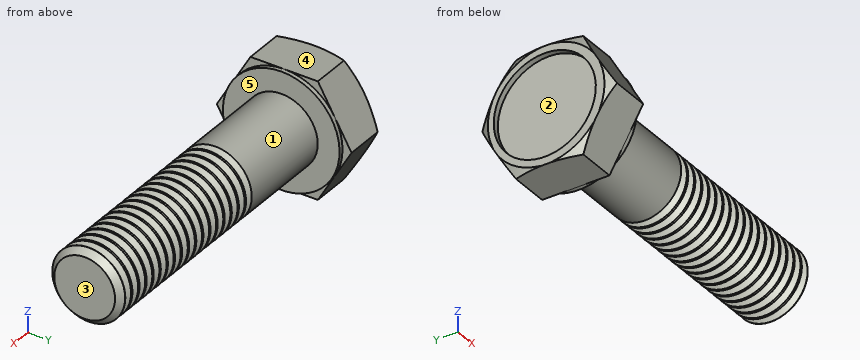
```python
from build123d import *

# Parameters (mm, degrees)
BASEHEAD_DEPTH     = 6.63
INDENT_START       = -0.82875
INDENT_2_OUTLINE_R = 7
INDENT_2_DEPTH     = 0.82875
SKETCH4_W          = 0.6
SKETCH4_H          = 11.237604307
THDSCHPAT_COUNT    = 18
THDSCHPAT_PITCH    = 1.444444444


# Read off the part's stored shape, not the designer's step: Indent
with BuildPart() as part:
    # Sketch1 → BaseHead (new body)
    with BuildSketch(Plane(origin=(0, 0, 0), x_dir=(0, 0, -1), z_dir=(1, 0, 0))):
        Polygon((8, 4.618802154), (8, -4.618802154), (0, -9.237604307), (-8, -4.618802154), (-8, 4.618802154), (0, 9.237604307), align=None)
    extrude(amount=BASEHEAD_DEPTH)

    # Indent outline → Indent (revolve)
    with BuildSketch(Plane.YX):
        Polygon((5, 6.63), (5, 45.802), (4.172, 46.63), (0, 46.63), (0, 6.63), align=None)
    revolve(axis=Axis((0, 0, 0), (1, 0, 0)))

    # Indent 2 outline → Indent 2 (cut)
    with BuildSketch(Plane.ZY.offset(INDENT_START)):
        with Locations((0.033212245, 0.192376607)):
            Circle(INDENT_2_OUTLINE_R)
    extrude(amount=INDENT_2_DEPTH, mode=Mode.SUBTRACT)

    # Sketch3 → HeadChamfer (revolve, cut)
    with BuildSketch(Plane.XY, mode=Mode.PRIVATE) as headchamfer_sk:
        Polygon((0, 8), (3.601282526, 14.237604307), (3.601282526, 19.237604307), (-10, 19.237604307), (-10, 8), align=None)
    revolve(headchamfer_sk.sketch.rotate(Axis((0, 0, 0), (1, 0, 0)), 90), axis=Axis((0, 0, 0), (1, 0, 0)), mode=Mode.SUBTRACT)

    # Sketch4 → BearingFace (revolve, cut)
    with BuildSketch(Plane.XY, mode=Mode.PRIVATE) as bearingface_sk:
        with Locations((6.33, 13.618802154)):
            Rectangle(SKETCH4_W, SKETCH4_H)
    revolve(bearingface_sk.sketch.rotate(Axis((0, 0, 0), (1, 0, 0)), 90), axis=Axis((0, 0, 0), (1, 0, 0)), mode=Mode.SUBTRACT)

    # ThdSchSke → ThreadSchematic (revolve, cut)
    with BuildSketch(Plane.XY):
        Polygon((20.63, -4.172), (20.050228158, -5), (20.050228158, -6.25), (21.209771842, -6.25), (21.209771842, -5), align=None)
    threadschematic = revolve(axis=Axis((-3.175, 0, 0), (1, 0, 0)), mode=Mode.SUBTRACT)

    # ThdSchPat: ThreadSchematic ×18
    with Locations(*[(i * THDSCHPAT_PITCH, 0, 0) for i in range(1, THDSCHPAT_COUNT)]):
        add(threadschematic, mode=Mode.SUBTRACT)


solid = part.part
```
Build history of the part. All positions in model axes, mm. Face numbers are marked on the shaded views. A direction names the side the tool comes from. Coordinates: 2 decimals unless noted, no trailing zeros. Order: outer loops, then holes, each group sorted by start corner. A loop starts at its lowest first (then second) coordinate and runs counter-clockwise, first axis right, second up. Notation, with made-up numbers: M 51.25,81 L 109.25,81 A18 ccw 109.25,90 Z; hole C 30,24 d6. An arc over 180 degrees is marked long. One line per question, with ' | ' between items. Start each with the question number.
1. Cut at A-A (x = 13.5). Write the cut outline in (y, z).
2. Tool access for the marked faces 4 and 5: list every direction of +Z, -Z, +X, -X, +Y, -Y with a clear straight run to the whole face (end or side of a thin tool).
3. Wall check: line 1 along X through (y, z) = (-6, -0.5); line 2 along X through (y, z) = (1, -0.25); line 3 along Y through (x, z) = (19, 0.5). Give the ranges that are in metal, low to high. Write a range as [from, to].
4. Mould opens along Z. For the marked faces 1, 2 and 3 say: +Z half, -Z half, draft (parallel to the pull), parting line (faces both ways), or undercut.
5. Flat gauge pins, fed straight in: P1, Ø3, axis at y = 4.5, z = 6.5, coming from the +X side; P2, Ø5, axis at x = 41.5, y = 3, coming from the +Z side; P3, Ø4, axis at x = 25, z = 0, coming from the -Y side. Where does each tip first touch, or does it go through?
The answers:
1) outline: C 0,0 d10
2) face 4: +Z, +X, -X, +Y, -Y | face 5: +X
3) line 1: x = [0.83, 6.63] | line 2: x = [0.83, 46.63] | line 3: y = [-4.97, 4.97]
4) face 1: parting line | face 2: undercut | face 3: draft
5) P1: stops at x = 6.63 | P2: stops at z = 4.97 | P3: stops at y = -5
